Job drawing, mm, ordinate dimensions from the low corner. One solid piece. A direction names the side the tool comes from. Give positions to 0.01 mm unless a question says otherwise; leave off trailing zeros. Order: outer loops, then holes, each group sorted by start corner. A loop starts at its lowest first (then second) coordinate and runs counter-clockwise, first axis right, second up. Notation, with made-up numbers: M 78,63 L 126,63 A20 ccw 126,76 Z; hole C 31,-8.75 d8. An arc over 180 degrees is marked long. Put each result on its own line as item: value. Start each with the question number.
1) Cut at C-C (z = 3.9). Write the cut outline in (x, y).
2) Pin check, flat tips, straight feed: pin 1 (8 mm diameter, centred on y = 20.5, z = 59.5, fed in from +X); pin 2 (11 mm diameter, centred on x = 4, z = 58.5, fed in from +Y); pin 3 (5 mm diameter, centred on x = 67, y = 6, fed in from -Z). Stop position of each tip, or through.
3) Two-plate mould, pull along X, no slides. Class the marked faces 1, 2 and 3: released by +X, released by -X, zero draft, split by the parting line, or undercut.
4) Cut at A-A (y = 21.5). Write the cut outline in (x, z).
5) Tool access for the marked faces 4, 5 and 6: list every direction of +Z, -Z, +X, -X, +Y, -Y with a clear straight run to the whole face (end or side of a thin tool).
6) Cut at B-B (x = 35.5). Write the cut outline in (y, z), and give its area (3 significant figures).
7) Cut at D-D (y = 5). Write the cut outline in (x, z).
8) Drill centre lines: line 1 (X direction, y = 19, z = 19); line 2 (Y direction, x = 5, z = 51); line 3 (X direction, y = 7.25, z = 78.1). Where is each one in solid material? Low to high. Write a range as [from, to].
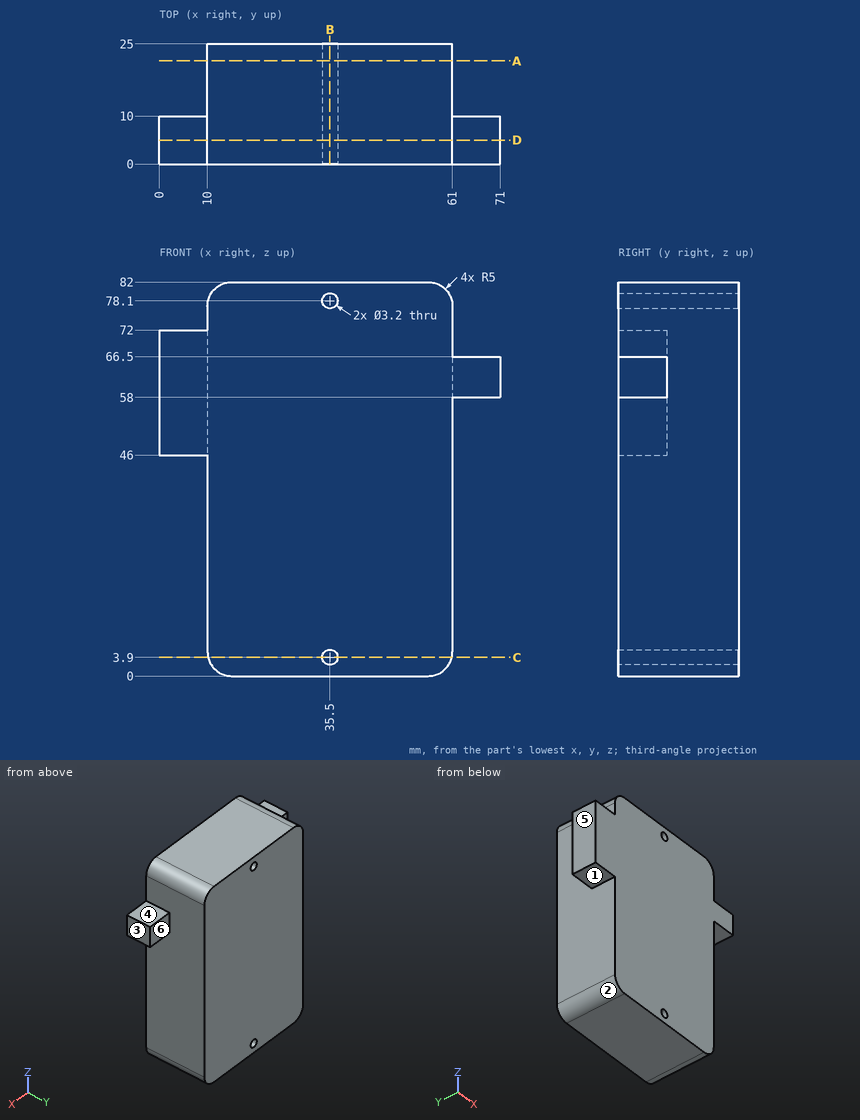
Solution:
1. outline: M 10.12,0 L 33.9,0 L 33.9,25 L 10.12,25 Z; M 37.1,0 L 60.88,0 L 60.88,25 L 37.1,25 Z
2. pin 1: x = 61
2. pin 2: y = 10
2. pin 3: z = 58
3. face 1: zero draft
3. face 2: released by -X
3. face 3: released by +X
4. outline: M 10,5 A5 ccw 15,0 L 56,0 A5 ccw 61,5 L 61,77 A5 ccw 56,82 L 15,82 A5 ccw 10,77 Z; hole C 35.5,3.9 d3.2; hole C 35.5,78.1 d3.2
5. face 4: +Z, +X, +Y, -Y
5. face 5: +Z, -Z, -X, +Y, -Y
5. face 6: +Z, -Z, +X, +Y
6. outline: M 0,0 L 25,0 L 25,2.3 L 0,2.3 Z; M 0,5.5 L 25,5.5 L 25,76.5 L 0,76.5 Z; M 0,79.7 L 25,79.7 L 25,82 L 0,82 Z
6. area: 1,890 mm²
7. outline: M 0,46 L 10,46 L 10,5 A5 ccw 15,0 L 56,0 A5 ccw 61,5 L 61,58 L 71,58 L 71,66.5 L 61,66.5 L 61,77 A5 ccw 56,82 L 15,82 A5 ccw 10,77 L 10,72 L 0,72 Z; hole C 35.5,3.9 d3.2; hole C 35.5,78.1 d3.2
8. line 1: [10, 61]
8. line 2: [0, 10]
8. line 3: [10.12, 33.9], [37.1, 60.88]
